from build123d import *

# Parameters (mm, degrees)
PAD_DEPTH       = 22
SKETCH001_R     = 4
POCKET_DEPTH    = 22
POCKET001_DEPTH = 10
SKETCH002_R     = 4.2
POCKET002_DEPTH = 22


with BuildPart() as part:
    # Sketch → Pad (new body)
    with BuildSketch(Plane.XY):
        with BuildLine():
            Line((-10, 10), (60, 10))
            Line((60, 10), (60, 0))
            ThreePointArc((45, -10), (54.013878, -7.270817), (60, 0))
            Line((10, -10), (45, -10))
            Line((10, -30), (10, -10))
            Line((-10, -30), (10, -30))
            Line((-10, 10), (-10, -30))
        make_face()
    extrude(amount=PAD_DEPTH)

    # Sketch001 → Pocket (cut)
    with BuildSketch(Plane.XY):
        with Locations((40, 0)):
            Circle(SKETCH001_R)
    extrude(amount=POCKET_DEPTH, mode=Mode.SUBTRACT)

    # Sketch004 → Pocket001 (cut)
    with BuildSketch(Plane.XY):
        with BuildLine():
            ThreePointArc((40, 11), (29, 0), (40, -11))
            Line((40, -11), (45, -11))
            ThreePointArc((45, -11), (54.340905, -7.958424), (60.1, 0))
            Line((60.1, 11), (60.1, 0))
            Line((40, 11), (60.1, 11))
        make_face()
    extrude(amount=POCKET001_DEPTH, mode=Mode.SUBTRACT)

    # Sketch002 → Pocket002 (cut)
    with BuildSketch(Plane.XY.offset(22)):
        Circle(SKETCH002_R)
    extrude(amount=-POCKET002_DEPTH, mode=Mode.SUBTRACT)


solid = part.part
Could you check a few things on this model? Use its own coordinates, in mm. A direction names the side the tool comes from. Coordinates: 2 decimals unless noted, no trailing zeros. Loops run counter-clockwise (first coordinate to the right, second up) from the corner with the lowest first, then second, coordinate; pieces in that order, holes last.
1. For faces 1 (the face through (10, -20, 11)), 2 (the face through (0, -30, 11)), 3 (the face through (29, 0, 5)), which set-ups out of +Z, -Z, +X, -X, +Y, -Y let a thin tool reach every point of the face, with its end or its side?
2. We'd pull the mould along Y, two halves only. Please class faces 4 (the face through (8, -5, 0)), 5 (the face through (4.006, 1.262, 11.154)), 6 (the face through (17, 10, 11)), 7 (the face through (44.3, 0.1, 10)): released by +Y, released by -Y, zero draft, split by the parting line, or undercut.
3. Imagine slicing it at A-A (x = 40). Please give me the cut outline in (y, z), and give its area (3 significant figures).
4. I need wall thicknesses on L1, parallel to Y at x = 40, z = 14.5; L2, parallel to Y at x = 0, z = 6; L3, parallel to X at y = -3, z = 17.75. Which ranges of each line are inside material? Lowest first, please.
5. Imagine slicing it at B-B (z = 13). Please give me the cut outline in (x, y), and give its area (3 significant figures).
6. For P1, Ø12, axis at x = 37, y = -14, coming from the -Z side; P2, Ø16, axis at x = 44.5, y = -2.5, coming from the -Z side; P3, Ø5, axis at x = 0, y = 0, coming from the +Z side, each with a flat end and sliding along its axis, tell me the tip position at first contact or that it passes through.
7. Imagine slicing it at C-C (y = 3). Please give me the cut outline in (x, z), and give its area (3 significant figures).
8. Imagine slicing it at D-D (z = 6.25). Please give me the cut outline in (x, y), and give its area (3 significant figures).
Computed values:
1. face 1: +Z, -Z, +X, -Y
1. face 2: +Z, -Z, +X, -X, -Y
1. face 3: -Z, +X
2. face 4: zero draft
2. face 5: undercut
2. face 6: released by +Y
2. face 7: undercut
3. outline: (-10, 10) - (-4, 10) - (-4, 22) - (-10, 22) - close; (4, 10) - (10, 10) - (10, 22) - (4, 22) - close
3. area: 144 mm2
4. L1: y = -10 to -4, 4 to 10
4. L2: y = -30 to -4.2, 4.2 to 10
4. L3: x = -10 to -2.94, 2.94 to 37.35, 42.65 to 58.36
5. outline: (-10, -30) - (10, -30) - (10, -10) - (45, -10) arc R16.25 ccw to (60, 0) - (60, 10) - (-10, 10) - close; hole circle Ø8.4 at (0, 0); hole circle Ø8 at (40, 0)
5. area: 1,650 mm2
6. P1: stops at z = 0
6. P2: stops at z = 10
6. P3: passes through
7. outline: (-10, 0) - (-2.94, 0) - (-2.94, 22) - (-10, 22) - close; (2.94, 0) - (29.42, 0) - (29.42, 10) - (37.35, 10) - (37.35, 22) - (2.94, 22) - close; (42.65, 10) - (60, 10) - (60, 22) - (42.65, 22) - close
7. area: 1,040 mm2
8. outline: (-10, -30) - (10, -30) - (10, -10) - (35.42, -10) arc R11 cw to (35.42, 10) - (-10, 10) - close; hole circle Ø8.4 at (0, 0)
8. area: 1,160 mm2
